Design review of the part built by this model. Coordinates are the model's own, in mm. A direction names the side the tool comes from. Give positions to 0.01 mm unless a question says otherwise; leave off trailing zeros. Order: outer loops, then holes, each group sorted by start corner. A loop starts at its lowest first (then second) coordinate and runs counter-clockwise, first axis right, second up. Notation, with made-up numbers: (67, 62.25) -> (110, 62.25) arc R14 cw to (110, 84.25) -> close; hole circle Ø4 at (14, 76.25). An arc over 180 degrees is marked (long way). One line per item, written item: value. Start each with the question number.
1) Wall thickness on line 1 along Z through (x, y) = (8, 7.95); line 2 along Z through (x, y) = (76, 3.5); line 3 along X through (y, z) = (5.5, -8.5): over which ranges is each line inside the solid? List them lowest first. Write a range as from..to.
2) Consider section B-B (y = 1.75). State the section outline as (x, z) points, plus the area to 3 significant figures.
3) Tool access review of faces 4 (the face through (0, 5, -29)), 5 (the face through (70.505, 3.451, -7.758)): name each direction out of +Z, -Z, +X, -X, +Y, -Y from which nothing blocks a thin tool from reaching the whole face with its end or side.
4) For pin 1 (4 mm diameter, centred on x = 8, z = -50, fed in from -Y), flat-tipped, find the tip position at first contact; note if it passes through.
5) Consider section C-C (z = -8). State the section outline as (x, y) points, plus the area to 3 significant figures.
6) The part is to be moulded in two halves that separate along X. For faces 1 (the face through (41, 5, -58)), 2 (the face through (84, 5, -29)), 3 (the face through (8.46, 8.52, -46.53)), say which applies: released by +X, released by -X, zero draft, split by the parting line, or undercut.
7) Consider section A-A (x = 8). State the section outline as (y, z) points, plus the area to 3 significant figures.
from build123d import *

# Parameters (mm, degrees)
SKETCH1_W                                     = 84
SKETCH1_H                                     = 58
EXTRUDE1_DEPTH                                = 10
CBORE_FOR_M6_HEX_SOCKET_HEAD_CAP1_D           = 7
CBORE_FOR_M6_HEX_SOCKET_HEAD_CAP1_CBORE_D     = 11
CBORE_FOR_M6_HEX_SOCKET_HEAD_CAP1_CBORE_DEPTH = 7
LPATTERN1_COUNT                               = 2
LPATTERN1_PITCH                               = 68
LPATTERN1_COUNT_DIR2                          = 2
LPATTERN1_PITCH_DIR2                          = 42
FILLET1_R                                     = 4


with BuildPart() as part:
    # Sketch1 → Extrude1 (new body)
    with BuildSketch(Plane(origin=(0, 0, 0), x_dir=(1, 0, 0), z_dir=(0, 1, 0))):
        with Locations((42, 29)):
            Rectangle(SKETCH1_W, SKETCH1_H)
    extrude(amount=EXTRUDE1_DEPTH)

    # CBORE for M6 Hex Socket Head Cap1 (through all)
    with Locations(Plane.XZ):
        with Locations((76, -50)):
            cbore_for_m6_hex_socket_head_cap1 = CounterBoreHole(CBORE_FOR_M6_HEX_SOCKET_HEAD_CAP1_D / 2, CBORE_FOR_M6_HEX_SOCKET_HEAD_CAP1_CBORE_D / 2, CBORE_FOR_M6_HEX_SOCKET_HEAD_CAP1_CBORE_DEPTH)

    # LPattern1: CBORE for M6 Hex Socket Head Cap1 2 × 2
    with Locations(*[(-i * LPATTERN1_PITCH, 0, j * LPATTERN1_PITCH_DIR2) for i in range(LPATTERN1_COUNT) for j in range(LPATTERN1_COUNT_DIR2) if (i, j) != (0, 0)]):
        add(cbore_for_m6_hex_socket_head_cap1, mode=Mode.SUBTRACT)

    # Fillet1
    fillet1_edges = [part.edges().sort_by_distance(p)[0] for p in [
        (0, 5, -58),
        (84, 5, -58),
        (84, 5, 0),
        (0, 5, 0),
    ]]
    fillet(fillet1_edges, radius=FILLET1_R)


solid = part.part
Checked values:
1. line 1: z = -58..-53.5, -46.5..-11.5, -4.5..0
1. line 2: z = -58..-55.5, -44.5..-13.5, -2.5..0
1. line 3: x = 0..2.52, 13.48..70.52, 81.48..84
2. outline: (0, -54) arc R4 ccw to (4, -58) -> (80, -58) arc R4 ccw to (84, -54) -> (84, -4) arc R4 ccw to (80, 0) -> (4, 0) arc R4 ccw to (0, -4) -> close; hole circle Ø11 at (8, -50); hole circle Ø11 at (8, -8); hole circle Ø11 at (76, -50); hole circle Ø11 at (76, -8)
2. area: 4,480 mm^2
3. face 4: +Z, -Z, -X, +Y, -Y
3. face 5: -Y
4. pin 1: passes through
5. outline: (0, 0) -> (2.5, 0) -> (2.5, 7) -> (4.5, 7) -> (4.5, 10) -> (0, 10) -> close; (11.5, 7) -> (13.5, 7) -> (13.5, 0) -> (70.5, 0) -> (70.5, 7) -> (72.5, 7) -> (72.5, 10) -> (11.5, 10) -> close; (79.5, 7) -> (81.5, 7) -> (81.5, 0) -> (84, 0) -> (84, 10) -> (79.5, 10) -> close
5. area: 644 mm^2
6. face 1: zero draft
6. face 2: released by +X
6. face 3: undercut
7. outline: (0, -58) -> (10, -58) -> (10, -53.5) -> (7, -53.5) -> (7, -55.5) -> (0, -55.5) -> close; (0, -44.5) -> (7, -44.5) -> (7, -46.5) -> (10, -46.5) -> (10, -11.5) -> (7, -11.5) -> (7, -13.5) -> (0, -13.5) -> close; (0, -2.5) -> (7, -2.5) -> (7, -4.5) -> (10, -4.5) -> (10, 0) -> (0, 0) -> close
7. area: 384 mm^2
